Could you check a few things on this drawing? It's one solid part, dimensions in mm from its lowest x, y, z. A direction names the side the tool comes from. Give positions to 0.01 mm unless a question says otherwise; leave off trailing zeros. Loops run counter-clockwise (first coordinate to the right, second up) from the corner with the lowest first, then second, coordinate; pieces in that order, holes last. Notation, with made-up numbers: (73.5, -19) - (131.5, -19) arc R27 cw to (131.5, 15) - close; hole circle Ø2 at (23, 73.5). An arc over 180 degrees is marked (long way). Use CSV: the item, a comma, the result in double quotes.
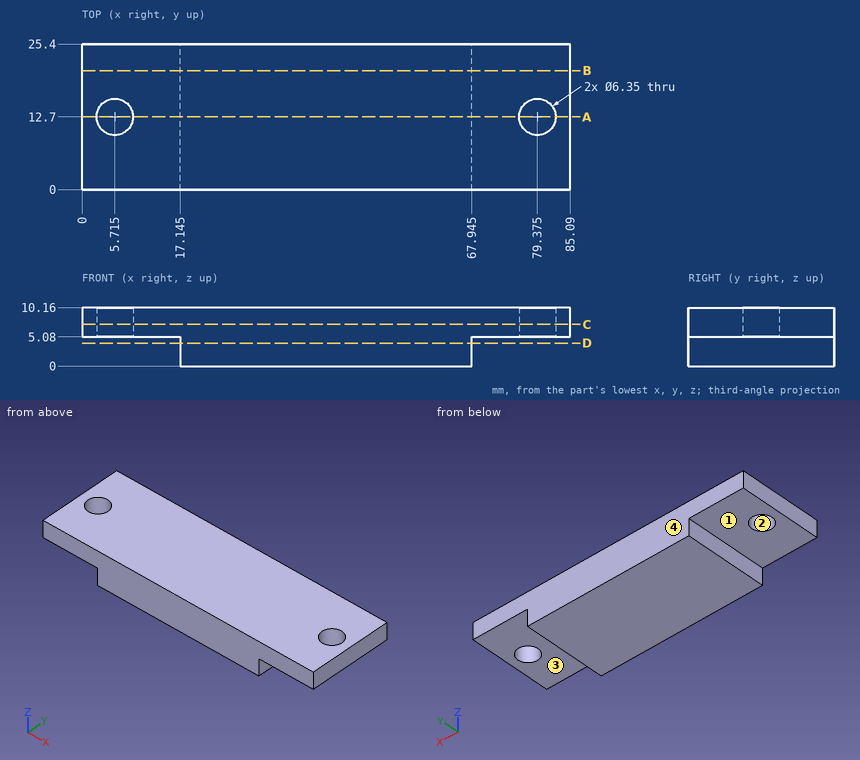
1) Suppose I cut it at D-D (z = 4). Please give me the cut outline in (x, y) (3 decimals), plus the area to 3 significant figures.
Answer below:
outline,"(17.145, 0) - (67.945, 0) - (67.945, 25.4) - (17.145, 25.4) - close"
area,"1,290 mm2"
2) I need wall thicknesses on line 1 along X through (y, z) = (1.5, 4) (3 decimals); line 2 along Y through (x, z) = (80, 7.25); line 3 along Z through (x, y) = (68, 13). Which ranges of each line are inside material? Lowest first, please.
Answer below:
line 1,"x = 17.145 to 67.945"
line 2,"y = 0 to 9.59, 15.81 to 25.4"
line 3,"z = 5.08 to 10.16"
3) Suppose I cut it at B-B (y = 20.75). Please give me the cut outline in (x, z) (3 decimals).
Answer below:
outline,"(0, 5.08) - (17.145, 5.08) - (17.145, 0) - (67.945, 0) - (67.945, 5.08) - (85.09, 5.08) - (85.09, 10.16) - (0, 10.16) - close"
4) I'm going to push flat-ended pins straight in: P1, Ø1, axis at y = 18, z = 2.5, coming from the +X side (3 decimals); P2, Ø1.5, axis at y = 17.5, z = 3.5, coming from the -X side (3 decimals); P3, Ø5, axis at x = 76.5, y = 13.5, coming from the -Z side; P4, Ø4, axis at x = 79.375, y = 12.7, coming from the -Z side. Where does each tip first touch, or does it pass through?
Answer below:
P1,"stops at x = 67.945"
P2,"stops at x = 17.145"
P3,"stops at z = 5.08"
P4,"passes through"
5) Suppose I cut it at C-C (z = 7.25). Please give me the cut outline in (x, y) (3 decimals).
Answer below:
outline,"(0, 0) - (85.09, 0) - (85.09, 25.4) - (0, 25.4) - close; hole circle Ø6.35 at (5.715, 12.7); hole circle Ø6.35 at (79.375, 12.7)"
6) Which directions (+Z, -Z, +X, -X, +Y, -Y) give clear straight access to the entire face, cutting with the end or side of a thin tool? Please do the marked faces 3 and 4.
Answer below:
face 3,"-Z, +X, +Y, -Y"
face 4,"+Z, -Z, +X, -X, +Y"
7) We'd pull the mould along X, two halves only. Please class the marked faces 1 and 2: +X half, -X half, draft (parallel to the pull), parting line (faces both ways), or undercut.
Answer below:
face 1,"draft"
face 2,"undercut"
8) Suppose I cut it at A-A (y = 12.7). Please give me the cut outline in (x, z) (3 decimals).
Answer below:
outline,"(0, 5.08) - (2.54, 5.08) - (2.54, 10.16) - (0, 10.16) - close; (8.89, 5.08) - (17.145, 5.08) - (17.145, 0) - (67.945, 0) - (67.945, 5.08) - (76.2, 5.08) - (76.2, 10.16) - (8.89, 10.16) - close; (82.55, 5.08) - (85.09, 5.08) - (85.09, 10.16) - (82.55, 10.16) - close"
